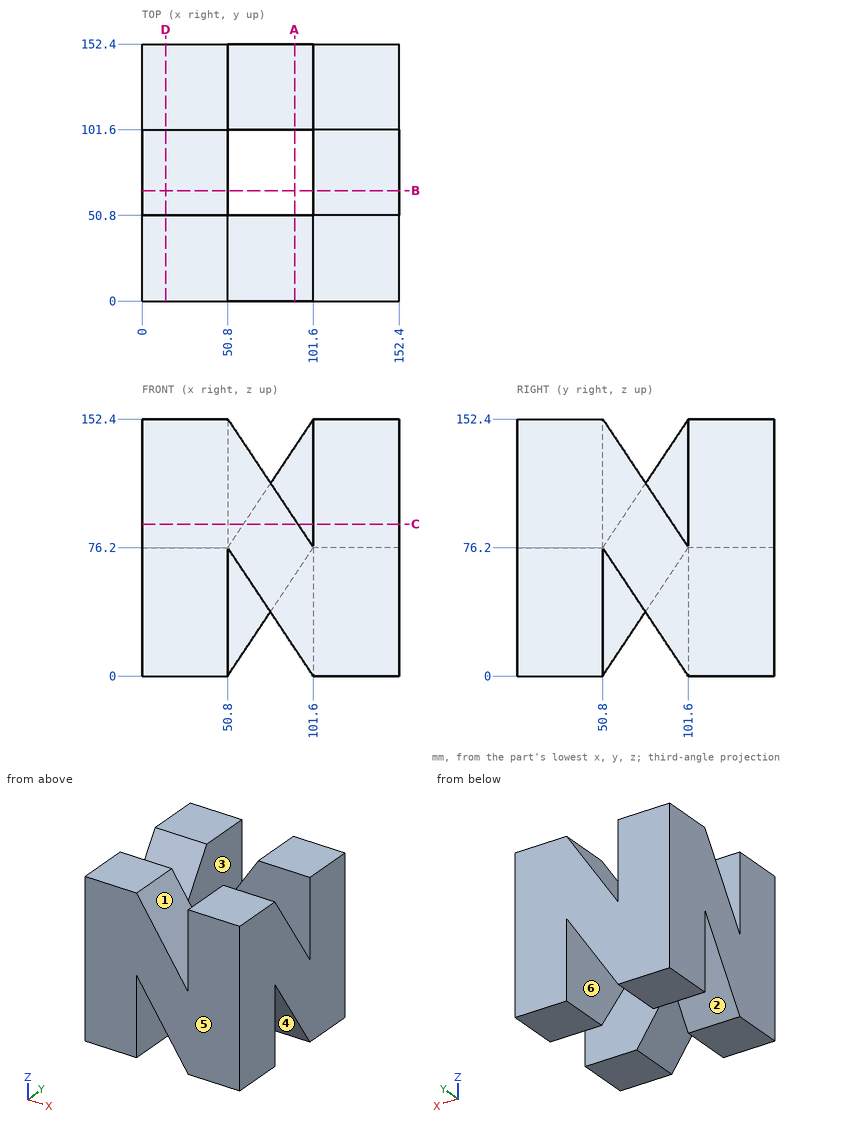
Check sheet for the drawn part. Datum: minimum x, y, z corner. Units: mm. A direction names the side the tool comes from. Give positions to 0.01 mm unless a question says otherwise; leave off trailing zeros. Order: outer loops, then holes, each group sorted by start corner. A loop starts at its lowest first (then second) coordinate and runs counter-clockwise, first axis right, second up. Notation, with made-up numbers: (-28, 27.5) - (18, 27.5) arc R23 ccw to (18, 48.5) - close; hole circle Ø5 at (76.5, 2). An arc over 180 degrees is marked (long way). Write item = value, one per line. Start each with the question number.
1) Section check A-A (x = 90.5). Enter the section's corners in (y, z).
2) Gauge pin test, flat ends, axial feed: pin 1 Ø1 at (y, z) = (90.5, 93.5) entering from +X; pin 2 Ø4 at (y, z) = (89, 107.5) entering from +X; pin 3 Ø8 at (x, y) = (65, 49.5) entering from +Z. Record the tip position at first contact, or that the pin passes through.
3) Section check D-D (x = 14). Enter the section's corners in (y, z).
4) Section check C-C (z = 90). Enter the section's corners in (x, y), then the cut area to 3 significant figures.
5) Scan lines: L1, parallel to Y at x = 91, z = 64.5; L2, parallel to Y at x = 83.5, z = 41; L3, parallel to Y at x = 120, z = 144.5. Record each from-to range of solid material in increasing order.
6) Access from +Z, -Z, +X, -X, +Y, -Y to the whole of each face (thin tool, end or side, straight path). Record for the marked faces 1, 2 and 3.
7) Section check B-B (y = 65.5). Enter the section's corners in (x, z).
8) Draft check along Y on the marked faces 4, 5 and 6. Enter one of: released by +Y, released by -Y, zero draft, split by the parting line, or undercut.
Geometry check:
q1.outline = (0, 16.65) - (50.8, 16.65) - (50.8, 92.85) - (0, 92.85) - close; (101.6, 59.55) - (152.4, 59.55) - (152.4, 135.75) - (101.6, 135.75) - close
q2.pin_1 = 152.4
q2.pin_2 = 50.8
q2.pin_3 = 137.1
q3.outline = (0, 0) - (50.8, 0) - (101.6, 76.2) - (101.6, 0) - (152.4, 0) - (152.4, 152.4) - (101.6, 152.4) - (50.8, 76.2) - (50.8, 152.4) - (0, 152.4) - close
q4.outline = (0, 0) - (92.4, 0) - (92.4, 50.8) - (0, 50.8) - close; (0, 60) - (50.8, 60) - (50.8, 152.4) - (0, 152.4) - close; (60, 101.6) - (152.4, 101.6) - (152.4, 152.4) - (60, 152.4) - close; (101.6, 0) - (152.4, 0) - (152.4, 92.4) - (101.6, 92.4) - close
q4.area = 18,800 mm2
q5.L1 = 0 to 50.8, 101.6 to 152.4
q5.L2 = 0 to 50.8
q5.L3 = 0 to 56.07, 101.6 to 152.4
q6.face_1 = +Z, -Y
q6.face_2 = -Z, -X
q6.face_3 = none
q7.outline = (0, 22.05) - (50.8, 22.05) - (50.8, 98.25) - (0, 98.25) - close; (101.6, 54.15) - (152.4, 54.15) - (152.4, 130.35) - (101.6, 130.35) - close
q8.face_4 = undercut
q8.face_5 = released by -Y
q8.face_6 = zero draft
